Geometry: final body of the model. Coordinates: model frame, mm. A direction names the side the tool comes from. Give positions to 0.01 mm unless a question says otherwise; leave off trailing zeros. Write each loop counter-clockwise with the first axis right and the second up, starting at its lowest first coordinate (ties: lowest second). Pieces come first, ordered by that corner, then holes. Notation, with made-up numbers: (21, -8.5) -> (42, -8.5) arc R22 ccw to (42, 17.5) -> close; hole circle Ø7 at (-12, 84.25). An arc over 180 degrees is marked (long way). Answer in a Markdown table with one row per item. Add a question column.
Item 1: First-contact query: P1, Ø1.6, axis at x = -9, y = 6, coming from the +Z side; P2, Ø10, axis at x = -15, y = 14, coming from the -Z side; P3, Ø0.5, axis at y = 4, z = -2, coming from the +X side; P4, Ø1, axis at x = -28, z = 0.5, coming from the +Y side. Flat tips, straight axial feed; report the tip coordinate or a pass-through.
Item 2: Draft query along Z for faces 1 (the flat face through (-39, 6.568, -1)), 2 (the flat face through (-16, 6, 1.194)), 3 (the flat face through (-7, 3.568, -1)), 4 (the flat face through (-17, 6, -3.806)). Return one class per face: +Z half, -Z half, draft (parallel to the pull), parting line (faces both ways), or undercut.
Item 3: Material intervals for probe 1 along Z at (x, y) = (-3, 5); probe 2 along Y at (x, z) = (-30, -0.75); probe 3 along X at (y, z) = (15.5, 1.5), sorted ascending. Write a range as from..to.
Item 4: Access query for faces 5 (the flat face through (16.6, 4.1, -2.306)), 6 (the flat face through (-42.648, 5, -1)), 7 (the flat face through (11, 25, 1)), 8 (the flat face through (-21, 7.305, -1)), 9 (the cylindrical face through (-38.266, 5.047, -1.006)). Directions: +Z, -Z, +X, -X, +Y, -Y. A direction counts if a zero-diameter tool reaches every point of the face in a straight line with its end or side. Return the directions, or none.
Item 5: Section query C-C on y = 21.5. Output: boundary loops of the cut face in (x, z).
Item 6: Section query B-B on x = -36.5. Output: boundary loops of the cut face in (y, z).
Item 7: Section query A-A on y = 5.75. Output: boundary loops of the cut face in (x, z), plus the area to 3 significant figures.
```python
from build123d import *

# Parameters (mm, degrees)
BOSS_EXTRUDE1_DEPTH     = 9
CUT_EXTRUDE1_DEPTH      = 6
SKETCH3_R               = 3.434986687
BOSS_EXTRUDE2_DEPTH     = 16
SKETCH4_R               = 2.872742527
BOSS_EXTRUDE3_DEPTH     = 2
BOSS_EXTRUDE3_TAPER     = 24
SKETCH5_R               = 0.3
BOSS_EXTRUDE4_DEPTH     = 2
SKETCH6_W               = 59.861841092
SKETCH6_H               = 3.567823601
CUT_EXTRUDE2_DEPTH      = 2.5
CUT_EXTRUDE2_DEPTH_BACK = 7.5
SKETCH7_R               = 1
CUT_EXTRUDE3_DEPTH      = 3
SKETCH8_W               = 2
SKETCH8_H               = 1
CUT_EXTRUDE4_DEPTH      = 10.0001


with BuildPart() as part:
    # Sketch1 → Boss-Extrude1 (new body)
    with BuildSketch(Plane(origin=(0, 0, 0), x_dir=(1, 0, 0), z_dir=(0, 1, 0))):
        with BuildLine():
            Line((-42.647872244, 3.806239173), (10.091469849, 3.806239173))
            ThreePointArc((10.091469849, 3.806239173), (17.213968848, 1.306239173), (10.091469849, -1.193760827))
            Line((10.091469849, -1.193760827), (-42.647872244, -1.193760827))
            Line((-42.647872244, -1.193760827), (-42.647872244, 3.806239173))
        make_face()
    extrude(amount=BOSS_EXTRUDE1_DEPTH)

    # Sketch2 → Cut-Extrude1 (cut)
    with BuildSketch(Plane.XY.offset(1.193760827)):
        Polygon((1.39800972, 7.304936762), (3.426580057, 9), (1.39800972, 9), (-42.647872244, 9), (-42.647872244, 7.304936762), align=None)
    extrude(amount=-CUT_EXTRUDE1_DEPTH, mode=Mode.SUBTRACT)

    # Sketch3 → Boss-Extrude2 (add)
    with BuildSketch(Plane(origin=(0, 9, 0), x_dir=(1, 0, 0), z_dir=(0, 1, 0))):
        with Locations((13.213968848, 1.306239173)):
            Circle(SKETCH3_R)
    extrude(amount=BOSS_EXTRUDE2_DEPTH)

    # Sketch4 → Boss-Extrude3 (add)
    with BuildSketch(Plane(origin=(0, 25, 0), x_dir=(1, 0, 0), z_dir=(0, 1, 0))):
        with Locations((13.213968848, 1.306239173)):
            Circle(SKETCH4_R)
    extrude(amount=BOSS_EXTRUDE3_DEPTH, taper=BOSS_EXTRUDE3_TAPER)

    # Sketch5 → Boss-Extrude4 (add)
    with BuildSketch(Plane(origin=(0, 27, 0), x_dir=(1, 0, 0), z_dir=(0, 1, 0))):
        with Locations((13.213968848, 1.306239173)):
            Circle(SKETCH5_R)
    extrude(amount=BOSS_EXTRUDE4_DEPTH)

    # Sketch6 → Cut-Extrude2 (cut, two sides)
    with BuildSketch(Plane.XY.offset(1.193760827)) as cut_extrude2_sk:
        with Locations((-12.716951698, 1.783911801)):
            Rectangle(SKETCH6_W, SKETCH6_H)
    extrude(amount=CUT_EXTRUDE2_DEPTH, mode=Mode.SUBTRACT)
    extrude(cut_extrude2_sk.sketch, amount=-CUT_EXTRUDE2_DEPTH_BACK, mode=Mode.SUBTRACT)

    # Sketch7 → Cut-Extrude3 (cut)
    with BuildSketch(Plane.XZ.offset(-3.567823601)):
        with Locations((-39.22011329, -1.306239173)):
            Circle(SKETCH7_R)
    extrude(amount=-CUT_EXTRUDE3_DEPTH, mode=Mode.SUBTRACT)

    # Sketch8 → Cut-Extrude4 (cut)
    with BuildSketch(Plane(origin=(26, 0, 0), x_dir=(0, 0, -1), z_dir=(1, 0, 0))):
        with Locations((1.306239173, 4.067823601)):
            Rectangle(SKETCH8_W, SKETCH8_H)
    extrude(amount=-CUT_EXTRUDE4_DEPTH, mode=Mode.SUBTRACT)


solid = part.part
```
Findings below:
| question | item | result |
|---|---|---|
| 1 | P1 | stops at z = 1.19 |
| 1 | P2 | passes through |
| 1 | P3 | stops at x = 16 |
| 1 | P4 | stops at y = 7.3 |
| 2 | face 1 | undercut |
| 2 | face 2 | +Z half |
| 2 | face 3 | draft |
| 2 | face 4 | -Z half |
| 3 | probe 1 | z = -3.81..1.19 |
| 3 | probe 2 | y = 3.57..7.3 |
| 3 | probe 3 | x = 11.23..15.19 |
| 4 | face 5 | +X, -Y |
| 4 | face 6 | +Z, -Z, -X, +Y, -Y |
| 4 | face 7 | +Y |
| 4 | face 8 | +Z, -Z, -X, +Y |
| 4 | face 9 | -Y |
| 5 | outline | circle Ø6.87 at (13.21, -1.31) |
| 6 | outline | (3.57, -3.81) -> (7.3, -3.81) -> (7.3, 1.19) -> (3.57, 1.19) -> close |
| 7 | outline | (-42.65, -3.81) -> (10.09, -3.81) arc R4 ccw (long way) to (10.09, 1.19) -> (-42.65, 1.19) -> close; hole circle Ø2 at (-39.22, -1.31) |
| 7 | area | 308 mm^2 |
